Verification items for the finished model (mm, model axes). Face numbers are marked on the shaded views. A direction names the side the tool comes from. Give positions to 0.01 mm unless a question says otherwise; leave off trailing zeros. Write each loop counter-clockwise with the first axis right and the second up, starting at its lowest first coordinate (ties: lowest second). Pieces come first, ordered by that corner, then holes. Notation, with made-up numbers: (4, 3) - (49, 3) arc R21 ccw to (49, 26) - close; hole circle Ø10 at (50.5, 19). An arc over 180 degrees is marked (long way). Answer as a JSON object with one key per item and string values. Group by question number.
Item 1: Go/stop test with flat-tipped pins: pin 1 (4 mm diameter, centred on y = 20, z = 1.5, fed in from -X); pin 2 (6 mm diameter, centred on y = 19, z = 7, fed in from +X). Record where each tip stops, or that it passes through.
Item 2: Sectioned sample at A-A, the plane x = 47.5. Record the boundary of the cut face in (y, z).
Item 3: Draft check along X on the marked faces 4, 5 and 6. Enter one of: +X half, -X half, draft (parallel to the pull), parting line (faces both ways), or undercut.
Item 4: Tool access check on the marked faces 1, 2 and 3. Record the directions out of +Z, -Z, +X, -X, +Y, -Y that give a thin tool (end or side, any length) a straight path to the whole face; none if there is none.
Item 5: Scan lines: line 1 along Y through (x, z) = (29, 3.75); line 2 along X through (y, z) = (-20, 8.5). Record each from-to range of solid material in increasing order. Write a range as [from, to].
Item 6: Sectioned sample at B-B, the plane y = -29. Record the boundary of the cut face in (x, z).
Item 7: Sectioned sample at D-D, the plane y = 5.5. Record the boundary of the cut face in (x, z).
```python
from build123d import *

# Parameters (mm, degrees)
SKETCH1_R               = 7.5
SKETCH1_R_2             = 1.5
SKETCH1_R_3             = 2.5
BOSS_EXTRUDE1_DEPTH     = 12
CUT_EXTRUDE1_DEPTH      = 74.10266753
CUT_EXTRUDE1_DEPTH_BACK = 74.10266753


with BuildPart() as part:
    # Sketch1 → Boss-Extrude1 (new body)
    with BuildSketch(Plane.XY):
        with BuildLine():
            Line((-56.464466094, 12.5), (-41.75, 12.5))
            ThreePointArc((-41.75, 12.5), (-40.512563133, 13.012563133), (-40, 14.25))
            Line((-40, 14.25), (-40, 34))
            ThreePointArc((-40, 34), (-38.242640687, 38.242640687), (-34, 40))
            Line((-34, 40), (34, 40))
            ThreePointArc((34, 40), (38.242640687, 38.242640687), (40, 34))
            Line((40, 34), (40, 14.25))
            ThreePointArc((40, 14.25), (40.512563133, 13.012563133), (41.75, 12.5))
            Line((41.75, 12.5), (56.464466094, 12.5))
            Line((56.464466094, 12.5), (60, 8.964466094))
            Line((60, 8.964466094), (60, -8.964466094))
            Line((60, -8.964466094), (56.464466094, -12.5))
            Line((56.464466094, -12.5), (41.75, -12.5))
            ThreePointArc((41.75, -12.5), (40.512563133, -13.012563133), (40, -14.25))
            Line((40, -14.25), (40, -34))
            ThreePointArc((40, -34), (38.242640687, -38.242640687), (34, -40))
            Line((34, -40), (-34, -40))
            ThreePointArc((-34, -40), (-38.242640687, -38.242640687), (-40, -34))
            Line((-40, -34), (-40, -14.25))
            ThreePointArc((-40, -14.25), (-40.512563133, -13.012563133), (-41.75, -12.5))
            Line((-41.75, -12.5), (-56.464466094, -12.5))
            Line((-56.464466094, -12.5), (-60, -8.964466094))
            Line((-60, -8.964466094), (-60, 8.964466094))
            Line((-60, 8.964466094), (-56.464466094, 12.5))
        make_face()
        with Locations((-47.5, 0)):
            Circle(SKETCH1_R, mode=Mode.SUBTRACT)
        with Locations(Location((47.5, 0, 0), (0, 0, 180))):
            Circle(SKETCH1_R, mode=Mode.SUBTRACT)
        with Locations((-55.985281374, 8.485281374)):
            Circle(SKETCH1_R_2, mode=Mode.SUBTRACT)
        with Locations((-39.014718626, -8.485281374)):
            Circle(SKETCH1_R_2, mode=Mode.SUBTRACT)
        with Locations((-39.014718626, 8.485281374)):
            Circle(SKETCH1_R_2, mode=Mode.SUBTRACT)
        with Locations((-55.985281374, -8.485281374)):
            Circle(SKETCH1_R_2, mode=Mode.SUBTRACT)
        with Locations(Location((39.014718626, -8.485281374, 0), (0, 0, 180))):
            Circle(SKETCH1_R_2, mode=Mode.SUBTRACT)
        with Locations(Location((55.985281374, -8.485281374, 0), (0, 0, 180))):
            Circle(SKETCH1_R_2, mode=Mode.SUBTRACT)
        with Locations(Location((55.985281374, 8.485281374, 0), (0, 0, 180))):
            Circle(SKETCH1_R_2, mode=Mode.SUBTRACT)
        with Locations(Location((39.014718626, 8.485281374, 0), (0, 0, 180))):
            Circle(SKETCH1_R_2, mode=Mode.SUBTRACT)
        with Locations((-29, 29)):
            Circle(SKETCH1_R_3, mode=Mode.SUBTRACT)
        with Locations(Location((29, 29, 0), (0, 0, 180))):
            Circle(SKETCH1_R_3, mode=Mode.SUBTRACT)
        with Locations((29, -29)):
            Circle(SKETCH1_R_3, mode=Mode.SUBTRACT)
        with Locations(Location((-29, -29, 0), (0, 0, 180))):
            Circle(SKETCH1_R_3, mode=Mode.SUBTRACT)
    extrude(amount=BOSS_EXTRUDE1_DEPTH)

    # Sketch2 → Cut-Extrude1 (cut, two sides: drawn at the far end of the back side and taken through both)
    with BuildSketch(Plane.XY.offset(12).offset(-CUT_EXTRUDE1_DEPTH_BACK)):
        with BuildLine():
            Line((-21.5, 27.5), (21.5, 27.5))
            ThreePointArc((21.5, 27.5), (25.742640687, 25.742640687), (27.5, 21.5))
            Line((27.5, 21.5), (27.5, -21.5))
            ThreePointArc((27.5, -21.5), (25.742640687, -25.742640687), (21.5, -27.5))
            Line((21.5, -27.5), (-21.5, -27.5))
            ThreePointArc((-21.5, -27.5), (-25.742640687, -25.742640687), (-27.5, -21.5))
            Line((-27.5, -21.5), (-27.5, 21.5))
            ThreePointArc((-27.5, 21.5), (-25.742640687, 25.742640687), (-21.5, 27.5))
        make_face()
    extrude(amount=CUT_EXTRUDE1_DEPTH + CUT_EXTRUDE1_DEPTH_BACK, mode=Mode.SUBTRACT)


solid = part.part
```
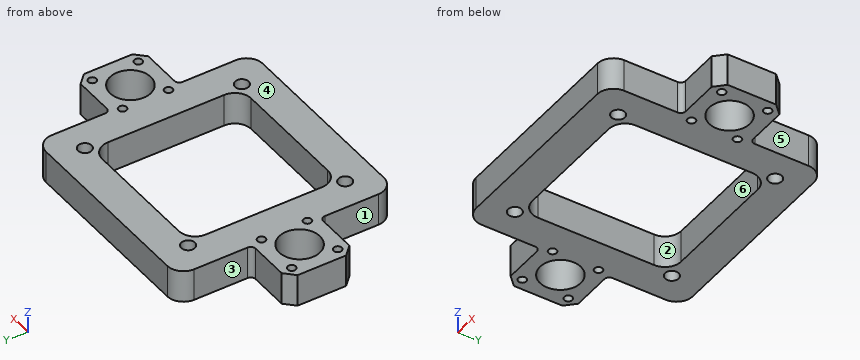
Geometry check:
{
 "1": {"pin 1": "x = -40", "pin 2": "x = 40"},
 "2": {"outline": "(-12.5, 0) - (-7.5, 0) - (-7.5, 12) - (-12.5, 12) - close; (7.5, 0) - (12.5, 0) - (12.5, 12) - (7.5, 12) - close"},
 "3": {"face 4": "draft", "face 5": "+X half", "face 6": "undercut"},
 "4": {"face 1": "+Z, -Z, -X, -Y", "face 2": "+Z, -Z", "face 3": "+Z, -Z, -X, +Y"},
 "5": {"line 1": "[-40, -31.5], [-26.5, 26.5], [31.5, 40]", "line 2": "[-40, -27.5], [27.5, 40]"},
 "6": {"outline": "(-40, 0) - (-31.5, 0) - (-31.5, 12) - (-40, 12) - close; (-26.5, 0) - (26.5, 0) - (26.5, 12) - (-26.5, 12) - close; (31.5, 0) - (40, 0) - (40, 12) - (31.5, 12) - close"},
 "7": {"outline": "(-60, 0) - (-52.6, 0) - (-52.6, 12) - (-60, 12) - close; (-42.4, 0) - (-27.5, 0) - (-27.5, 12) - (-42.4, 12) - close; (27.5, 0) - (42.4, 0) - (42.4, 12) - (27.5, 12) - close; (52.6, 0) - (60, 0) - (60, 12) - (52.6, 12) - close"}
}
